Autodesk Inventor part; units mm, degrees
ref_plane "YZ Plane" through (0, 0, 0) normal (1, 0, 0) x (0, 1, 0)
ref_plane "XZ Plane" through (0, 0, 0) normal (0, 1, 0) x (-1, 0, 0)
ref_plane "XY Plane" through (0, 0, 0) normal (0, 0, 1) x (1, 0, 0)
sketch "スケッチ1" plane through (0, 0, 0) normal (0, 0, 1) x (1, 0, 0)
  line L0 (-20, 20) -> (20, 20)
  line L1 (20, 20) -> (20, -20)
  line L2 (20, -20) -> (-20, -20)
  line L3 (-20, -20) -> (-20, 20)
  line L4 (-20, 20) -> (20, -20) construction
  line L5 (20, 20) -> (-20, -20) construction
  point P0 (0, 0)
  dimension "d0" = 40
  dimension "d1" = 40
extrude "押し出し1" add sketch "スケッチ1" along normal blind 1
sketch "スケッチ2" plane through (0, 0, 1) normal (0, 0, 1) x (1, 0, 0)
  line L0 (-20, 20) -> (-20, -20)
  line L1 (20, -20) -> (20, 20)
  line L2 (-20, -20) -> (20, -20)
  circle A0 centre (-10, -14) radius 1.55
  circle A1 centre (10, -14) radius 1.55
  point P0 (0, 0)
  dimension "d4" = 10
  dimension "d5" = 10
  dimension "d6" = 6
  dimension "d7" = 6
  dimension "d8" = 3.1
  dimension "d9" = 3.1
extrude "押し出し2" cut sketch "スケッチ2" against normal blind 1
sketch "スケッチ3" plane through (0, 0, 1) normal (0, 0, 1) x (1, 0, 0)
  line L0 (-20, 20) -> (20, 20)
  line L1 (20, 20) -> (20, 10)
  line L2 (20, 10) -> (-20, 10)
  line L3 (-20, 10) -> (-20, 20)
  line L4 (20, -20) -> (20, 20)
  line L5 (20, 20) -> (-20, 20)
  point P0 (0, 0)
  dimension "d12" = 40
  dimension "d13" = 10
  dimension "d14" = 0
  dimension "d15" = 0
extrude "押し出し3" cut sketch "スケッチ3" against normal blind 1
properties part number "gard"
The model under review builds one solid part; all positions refer to its coordinate system, in mm. Round coordinates to 2 decimals unless told otherwise and drop trailing zeros. Loops run counter-clockwise (first coordinate to the right, second up) from the corner with the lowest first, then second, coordinate; pieces in that order, holes last. Notation, with made-up numbers: (77, 44.25) -> (86, 44.25) arc R28 ccw to (86, 80.25) -> close; hole circle Ø10 at (-2, 63.5). An arc over 180 degrees is marked (long way). Answer as CSV lines item,"result".
1) Draft analysis for pull direction Y (two halves, no side actions). For faces 1 (the face through (9.798, -12.463, 0.507)), 2 (the face through (20, -4.8, 0.5)), 3 (the face through (0.3, 10, 0.5)), state which applies: pulls with the +Y half, pulls with the -Y half, needs draft (parallel to the pull), parting line crosses it, or undercut.
Geometry results:
face 1,"undercut"
face 2,"needs draft"
face 3,"pulls with the +Y half"
2) For P1, Ø1.5, axis at x = -9, y = -13.5, coming from the -Z side; P2, Ø2.5, axis at x = -10, y = -14, coming from the +Z side, all flat-tipped, find the tip position at first contact; note any pin that passes through.
Geometry results:
P1,"stops at z = 0"
P2,"passes through"
3) To check wall thickness, follow line 1 along Y through (x, z) = (-10, 0.7); line 2 along X through (y, z) = (-13.5, 0.8); line 3 along Y through (x, z) = (11, 0.55). State the ranges of each line that lie inside material, in increasing order. Write a range as from..to.
Geometry results:
line 1,"y = -20..-15.55, -12.45..10"
line 2,"x = -20..-11.47, -8.53..8.53, 11.47..20"
line 3,"y = -20..-15.18, -12.82..10"
4) Add section B-B on y = -14. Write out the cut boundary in (x, z), plus the area to 3 significant figures.
Geometry results:
outline,"(-20, 0) -> (-11.55, 0) -> (-11.55, 1) -> (-20, 1) -> close; (-8.45, 0) -> (8.45, 0) -> (8.45, 1) -> (-8.45, 1) -> close; (11.55, 0) -> (20, 0) -> (20, 1) -> (11.55, 1) -> close"
area,"33.8 mm²"
5) Add section A-A on x = 10. Write out the cut boundary in (y, z).
Geometry results:
outline,"(-20, 0) -> (-15.55, 0) -> (-15.55, 1) -> (-20, 1) -> close; (-12.45, 0) -> (10, 0) -> (10, 1) -> (-12.45, 1) -> close"
